```python
from build123d import *

# Parameters (mm, degrees)
BOSS_EXTRUDE1_DEPTH         = 12
M3_TAPPED_HOLE1_D           = 2.5
M3_TAPPED_HOLE1_DEPTH       = 7.5
M3_TAPPED_HOLE1_CSINK_D     = 3.05
M3_TAPPED_HOLE1_CSINK_ANGLE = 90
M3_TAPPED_HOLE1_TIP         = 0.751075774
M3_TAPPED_HOLE2_D           = 2.5
M3_TAPPED_HOLE2_DEPTH       = 7.5
M3_TAPPED_HOLE2_CSINK_D     = 3.05
M3_TAPPED_HOLE2_CSINK_ANGLE = 90
M3_TAPPED_HOLE2_TIP         = 0.751075774


with BuildPart() as part:
    # Sketch1 → Boss-Extrude1 (new body)
    with BuildSketch(Plane(origin=(0, 0, 0), x_dir=(1, 0, 0), z_dir=(0, 1, 0))):
        Polygon((-2.5, 1.443375673), (-2.5, -1.443375673), (0, -2.886751346), (2.5, -1.443375673), (2.5, 1.443375673), (0, 2.886751346), align=None)
    extrude(amount=BOSS_EXTRUDE1_DEPTH)

    # M3 Tapped Hole1
    with Locations(Plane(origin=(0, 12, 0), x_dir=(1, 0, 0), z_dir=(0, 1, 0))):
        with Locations((0, 0)):
            CounterSinkHole(M3_TAPPED_HOLE1_D / 2, M3_TAPPED_HOLE1_CSINK_D / 2, depth=M3_TAPPED_HOLE1_DEPTH, counter_sink_angle=M3_TAPPED_HOLE1_CSINK_ANGLE)
            with Locations((0, 0, -(M3_TAPPED_HOLE1_DEPTH + M3_TAPPED_HOLE1_TIP / 2))):  # 118° drill point
                Cone(0, M3_TAPPED_HOLE1_D / 2, M3_TAPPED_HOLE1_TIP, mode=Mode.SUBTRACT)

    # M3 Tapped Hole2
    with Locations(Plane(origin=(0, 0, 0), x_dir=(-1, 0, 0), z_dir=(0, -1, 0))):
        with Locations((0, 0)):
            CounterSinkHole(M3_TAPPED_HOLE2_D / 2, M3_TAPPED_HOLE2_CSINK_D / 2, depth=M3_TAPPED_HOLE2_DEPTH, counter_sink_angle=M3_TAPPED_HOLE2_CSINK_ANGLE)
            with Locations((0, 0, -(M3_TAPPED_HOLE2_DEPTH + M3_TAPPED_HOLE2_TIP / 2))):  # 118° drill point
                Cone(0, M3_TAPPED_HOLE2_D / 2, M3_TAPPED_HOLE2_TIP, mode=Mode.SUBTRACT)


solid = part.part
```
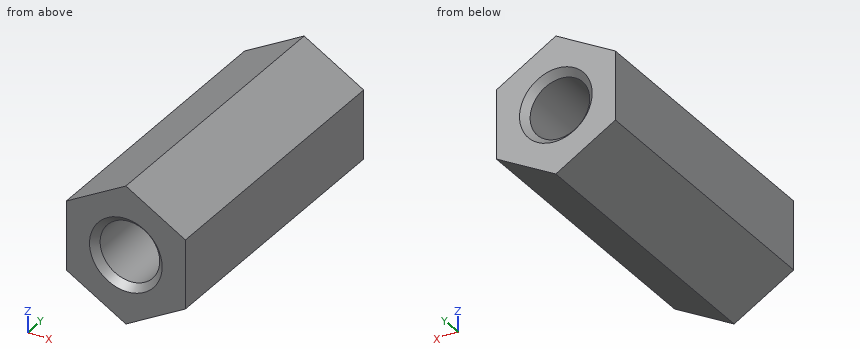
Geometry check sheet. Reference: the model listing, model coordinates, mm. Give positions to 0.01 mm unless a question says otherwise; leave off trailing zeros. Loops run counter-clockwise (first coordinate to the right, second up) from the corner with the lowest first, then second, coordinate; pieces in that order, holes last. Notation, with made-up numbers: (57, 38) - (68, 38) arc R11 cw to (68, 52) - close; hole circle Ø10 at (-29, 71.25). An arc over 180 degrees is marked (long way). Use CSV: the item, a comma, the result in double quotes. Start each with the question number.
Q1. Section check B-B, the plane x = 1.85. Record the cut outline in (y, z), and give its area (3 significant figures).
Q2. Go/stop test with flat-tipped pins: pin 1 Ø3 at (x, z) = (0, 0) entering from +Y (3 decimals); pin 2 Ø3 at (x, z) = (0, 0) entering from -Y (3 decimals). Record where each tip stops, or that it passes through.
Q3. Scan lines: probe 1 along X at (y, z) = (0.75, -0.2); probe 2 along X at (y, z) = (8.25, -0.95); probe 3 along Z at (x, y) = (0.9, 7.25). Record each from-to range of solid material in increasing order. Write a range as from..to.
Q4. Section check A-A, the plane y = 4.75. Record the cut outline in (x, z), and give its area (3 significant figures).
Q5. Section check C-C, the plane z = 2.5. Record the cut outline in (x, y).
Findings below:
1,outline,"(0, -1.82) - (12, -1.82) - (12, 1.82) - (0, 1.82) - close"
1,area,"43.6 mm^2"
2,pin 1,"stops at y = 11.975"
2,pin 2,"stops at y = 0.025"
3,probe 1,"x = -2.5..-1.23, 1.23..2.5"
3,probe 2,"x = -2.5..-0.81, 0.81..2.5"
3,probe 3,"z = -2.37..-0.87, 0.87..2.37"
4,outline,"(-2.5, -1.44) - (0, -2.89) - (2.5, -1.44) - (2.5, 1.44) - (0, 2.89) - (-2.5, 1.44) - close; hole circle Ø2.5 at (0, 0)"
4,area,"16.7 mm^2"
5,outline,"(-0.67, 0) - (0.67, 0) - (0.67, 12) - (-0.67, 12) - close"
